Work out the finished part from the listing and answer in its coordinate system (mm). A direction names the side the tool comes from. Give positions to 0.01 mm unless a question says otherwise; leave off trailing zeros. Order: outer loops, then holes, each group sorted by start corner. A loop starts at its lowest first (then second) coordinate and runs counter-clockwise, first axis right, second up.
```python
from build123d import *

# Parameters (mm, degrees)
SKETCH1_R           = 114.3
BOSS_EXTRUDE1_DEPTH = 12.7
SKETCH2_R           = 50.8
BOSS_EXTRUDE2_DEPTH = 25.4
SKETCH3_R           = 31.75
CUT_EXTRUDE1_DEPTH  = 118.11
SKETCH4_R           = 5
CUT_EXTRUDE2_DEPTH  = 118.11


with BuildPart() as part:
    # Sketch1 → Boss-Extrude1 (new body)
    with BuildSketch(Plane.XY):
        Circle(SKETCH1_R)
    extrude(amount=BOSS_EXTRUDE1_DEPTH)

    # Sketch2 → Boss-Extrude2 (add)
    with BuildSketch(Plane.XY.offset(12.7)):
        Circle(SKETCH2_R)
    extrude(amount=BOSS_EXTRUDE2_DEPTH)

    # Sketch3 → Cut-Extrude1 (cut)
    with BuildSketch(Plane.XY.offset(38.1)):
        Circle(SKETCH3_R)
    extrude(amount=-CUT_EXTRUDE1_DEPTH, mode=Mode.SUBTRACT)

    # Sketch4 → Cut-Extrude2 (cut)
    with BuildSketch(Plane.XY.offset(38.1)):
        with Locations((0, 41.275)):
            Circle(SKETCH4_R)
        with Locations((41.275, 0)):
            Circle(SKETCH4_R)
        with Locations((0, -41.275)):
            Circle(SKETCH4_R)
        with Locations((-41.275, 0)):
            Circle(SKETCH4_R)
    extrude(amount=-CUT_EXTRUDE2_DEPTH, mode=Mode.SUBTRACT)


solid = part.part
```
1. The part is cut by section D-D (z = 17). Write down the section's boundary in (x, y) (3 decimals).
Findings below:
outline: circle Ø101.6 at (0, 0); hole circle Ø10 at (-41.275, 0); hole circle Ø63.5 at (0, 0); hole circle Ø10 at (0, -41.275); hole circle Ø10 at (0, 41.275); hole circle Ø10 at (41.275, 0)
2. Straight lines are drawn through the part: probe 1 along Y at (x, z) = (0, 12) (3 decimals); probe 2 along Y at (x, z) = (4.5, 36); probe 3 along Z at (x, y) = (64, -57). For each, find the intervals that lie inside material, in ascending order.
Findings below:
probe 1: y = -114.3 to -46.275, -36.275 to -31.75, 31.75 to 36.275, 46.275 to 114.3
probe 2: y = -50.6 to -43.45, -39.1 to -31.43, 31.43 to 39.1, 43.45 to 50.6
probe 3: z = 0 to 12.7
3. Given P1, Ø6, axis at x = 8, z = 17, coming from the +Y side; P2, Ø3, axis at x = -76.5, z = 4.5, coming from the +Y side; P3, Ø5, axis at x = -69, y = 43, coming from the +Z side, each flat-ended and moving along its own axis, determine where each tip first touches the part or whether it passes through.
Findings below:
P1: stops at y = 50.55
P2: stops at y = 86.25
P3: stops at z = 12.7
4. Which of the six approach directions +Z, -Z, +X, -X, +Y, -Y give full straight-line access (tool end or side, diameter ignored) to faces 1 (the face through (49, -24, 12.7)), 2 (the face through (-1.084, 36.394, 19.317))?
Findings below:
face 1: +Z
face 2: +Z, -Z
5. The part is cut by section C-C (y = 27). Write down the section's boundary in (x, z).
Findings below:
outline: (-111.07, 0) - (-16.71, 0) - (-16.71, 38.1) - (-43.03, 38.1) - (-43.03, 12.7) - (-111.07, 12.7) - close; (16.71, 0) - (111.07, 0) - (111.07, 12.7) - (43.03, 12.7) - (43.03, 38.1) - (16.71, 38.1) - close
6. The mould has two halves that part along X. Classify faces 3 (the face through (-42.36, -4.88, 19.32)), 4 (the face through (24, -24, 0)), 5 (the face through (-114.19, 5.03, 6.26)): pulls with the +X half, pulls with the -X half, needs draft (parallel to the pull), parting line crosses it, or undercut.
Findings below:
face 3: undercut
face 4: needs draft
face 5: parting line crosses it
7. The part is cut by section A-A (x = 0). Write down the section's boundary in (y, z) (3 decimals), then the cut area to 3 significant figures.
Findings below:
outline: (-114.3, 0) - (-46.275, 0) - (-46.275, 38.1) - (-50.8, 38.1) - (-50.8, 12.7) - (-114.3, 12.7) - close; (-36.275, 0) - (-31.75, 0) - (-31.75, 38.1) - (-36.275, 38.1) - close; (31.75, 0) - (36.275, 0) - (36.275, 38.1) - (31.75, 38.1) - close; (46.275, 0) - (114.3, 0) - (114.3, 12.7) - (50.8, 12.7) - (50.8, 38.1) - (46.275, 38.1) - close
area: 2,300 mm2
